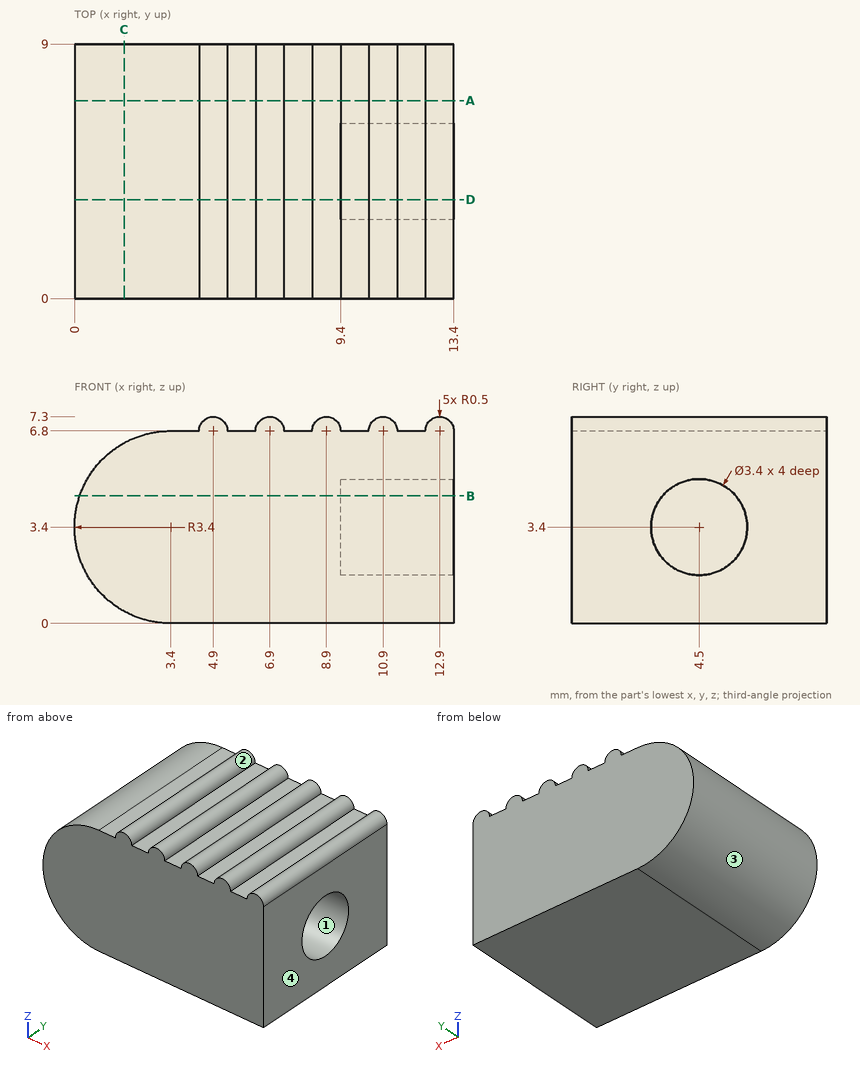
Input: dimensioned drawing with shaded views. Units: mm. Origin: part minimum x, y, z. Coordinates: 2 decimals unless noted, no trailing zeros. Order: outer loops, then holes, each group sorted by start corner. A loop starts at its lowest first (then second) coordinate and runs counter-clockwise, first axis right, second up. Notation, with made-up numbers: (-40, 45) -> (-16, 45) arc R10 cw to (-16, 50) -> close; hole circle Ø10 at (-39, -15). An arc over 180 degrees is marked (long way). Answer in a Markdown table with one row per item.
Item 1: Section C-C on x = 1.75. Output: boundary loops of the cut face in (y, z), plus the area to 3 significant figures.
Return value:
| item | result |
|---|---|
| outline | (0, 0.43) -> (9, 0.43) -> (9, 6.37) -> (0, 6.37) -> close |
| area | 53.5 mm² |
Item 2: Section B-B on z = 4.5. Output: boundary loops of the cut face in (x, y), plus the area to 3 significant figures.
Return value:
| item | result |
|---|---|
| outline | (0.18, 0) -> (13.4, 0) -> (13.4, 3.2) -> (9.4, 3.2) -> (9.4, 5.8) -> (13.4, 5.8) -> (13.4, 9) -> (0.18, 9) -> close |
| area | 109 mm² |
Item 3: Section D-D on y = 3.5. Output: boundary loops of the cut face in (x, z), plus the area to 3 significant figures.
Return value:
| item | result |
|---|---|
| outline | (3.4, 0) -> (13.4, 0) -> (13.4, 2.03) -> (9.4, 2.03) -> (9.4, 4.77) -> (13.4, 4.77) -> (13.4, 6.8) arc R0.5 ccw to (12.4, 6.8) -> (11.4, 6.8) arc R0.5 ccw to (10.4, 6.8) -> (9.4, 6.8) arc R0.5 ccw to (8.4, 6.8) -> (7.4, 6.8) arc R0.5 ccw to (6.4, 6.8) -> (5.4, 6.8) arc R0.5 ccw to (4.4, 6.8) -> (3.4, 6.8) arc R3.4 ccw to start |
| area | 77.1 mm² |
Item 4: Ray query, L1, parallel to Y at x = 12.25, z = 3.4; L2, parallel to Z at x = 11.9, y = 4.5; L3, parallel to Z at x = 10.9, y = 4.5. Return the intervals inside material, ascending.
Return value:
| item | result |
|---|---|
| L1 | y = 0 to 2.8, 6.2 to 9 |
| L2 | z = 0 to 1.7, 5.1 to 6.8 |
| L3 | z = 0 to 1.7, 5.1 to 7.3 |
Item 5: Draft query along Z for the marked faces 1, 2, 3 and 4. Return one class per face: released by +Z, released by -Z, zero draft, split by the parting line, or undercut.
Return value:
| item | result |
|---|---|
| face 1 | undercut |
| face 2 | released by +Z |
| face 3 | split by the parting line |
| face 4 | zero draft |
Item 6: Contact query for flat-ended pins moving along their axis: P1, Ø0.5, axis at x = 4, y = 6, coming from the +Z side; P2, Ø2, axis at y = 4.5, z = 3.4, coming from the +X side. Output: stop coordinate, or through.
Return value:
| item | result |
|---|---|
| P1 | stops at z = 6.8 |
| P2 | stops at x = 9.4 |
Item 7: Section A-A on y = 7. Output: boundary loops of the cut face in (x, z).
Return value:
| item | result |
|---|---|
| outline | (3.4, 0) -> (13.4, 0) -> (13.4, 6.8) arc R0.5 ccw to (12.4, 6.8) -> (11.4, 6.8) arc R0.5 ccw to (10.4, 6.8) -> (9.4, 6.8) arc R0.5 ccw to (8.4, 6.8) -> (7.4, 6.8) arc R0.5 ccw to (6.4, 6.8) -> (5.4, 6.8) arc R0.5 ccw to (4.4, 6.8) -> (3.4, 6.8) arc R3.4 ccw to start |
